```python
from build123d import *

# Parameters (mm, degrees)
SKETCH1_R           = 0.5
BOSS_EXTRUDE1_DEPTH = 3
SKETCH3_R           = 4.5
SKETCH3_R_2         = 2.5
BOSS_EXTRUDE2_DEPTH = 5
SKETCH4_R           = 3
CUT_EXTRUDE1_DEPTH  = 3


with BuildPart() as part:
    # Sketch1 → Boss-Extrude1 (new body)
    with BuildSketch(Plane(origin=(0, 0, 0), x_dir=(1, 0, 0), z_dir=(0, 1, 0))):
        with BuildLine():
            Line((0, 6.5), (29, 4))
            ThreePointArc((29, 4), (33, 0), (29, -4))
            Line((29, -4), (0, -6.5))
            ThreePointArc((0, -6.5), (-6.5, 0), (0, 6.5))
        make_face()
        with Locations(Location((14.5, 0, 0), (0, 0, 270))):
            Circle(SKETCH1_R, mode=Mode.SUBTRACT)
        with Locations(Location((17.5, 0, 0), (0, 0, 270))):
            Circle(SKETCH1_R, mode=Mode.SUBTRACT)
        with Locations(Location((20.5, 0, 0), (0, 0, 270))):
            Circle(SKETCH1_R, mode=Mode.SUBTRACT)
        with Locations(Location((23.5, 0, 0), (0, 0, 270))):
            Circle(SKETCH1_R, mode=Mode.SUBTRACT)
        with Locations(Location((26.5, 0, 0), (0, 0, 270))):
            Circle(SKETCH1_R, mode=Mode.SUBTRACT)
        with Locations(Location((29.5, 0, 0), (0, 0, 270))):
            Circle(SKETCH1_R, mode=Mode.SUBTRACT)
    extrude(amount=BOSS_EXTRUDE1_DEPTH)

    # Sketch3 → Boss-Extrude2 (add)
    with BuildSketch(Plane.XZ):
        with Locations(Location((0, 0, 0), (0, 0, 90))):
            Circle(SKETCH3_R)
        with Locations(Location((0, 0, 0), (0, 0, 270))):
            Circle(SKETCH3_R_2, mode=Mode.SUBTRACT)
    extrude(amount=BOSS_EXTRUDE2_DEPTH)

    # Sketch4 → Cut-Extrude1 (cut)
    with BuildSketch(Plane(origin=(0, 3, 0), x_dir=(1, 0, 0), z_dir=(0, 1, 0))):
        with Locations(Location((0, 0, 0), (0, 0, 270))):
            Circle(SKETCH4_R)
    extrude(amount=-CUT_EXTRUDE1_DEPTH, mode=Mode.SUBTRACT)


solid = part.part
```
Source: CAD feature listing. Evaluate the final solid. Frame: model axes, mm. A direction names the side the tool comes from. Coordinates: 2 decimals unless noted, no trailing zeros. Order: outer loops, then holes, each group sorted by start corner. A loop starts at its lowest first (then second) coordinate and runs counter-clockwise, first axis right, second up. Notation, with made-up numbers: (16.5, 79) - (70.5, 79) arc R18 ccw to (70.5, 97) - close; hole circle Ø3 at (55, 43.5). An arc over 180 degrees is marked (long way). One line per item, written item: value.
1) Contact query for flat-ended pins moving along their axis: pin 1 (2 mm diameter, centred on x = 21, y = 1, fed in from -Z); pin 2 (3 mm diameter, centred on y = -0.5, z = -2.5, fed in from +X); pin 3 (5.5 mm diameter, centred on x = 0, z = 0, fed in from +Y). Output: stop coordinate, or through.
Computed values:
pin 1: stops at z = -4.78
pin 2: stops at x = 32.85
pin 3: stops at y = 0
2) Cut plane B-B on y = 2. Output: boundary loops of the cut face in (x, z), plus the area to 3 significant figures.
Computed values:
outline: (0, -6.5) - (29, -4) arc R4 ccw to (29, 4) - (0, 6.5) arc R6.5 ccw to start; hole circle Ø6 at (0, 0); hole circle Ø1 at (14.5, 0); hole circle Ø1 at (17.5, 0); hole circle Ø1 at (20.5, 0); hole circle Ø1 at (23.5, 0); hole circle Ø1 at (26.5, 0); hole circle Ø1 at (29.5, 0)
area: 363 mm^2
3) Cut plane A-A on x = 14.5. Output: boundary loops of the cut face in (y, z).
Computed values:
outline: (0, -5.25) - (3, -5.25) - (3, -0.5) - (0, -0.5) - close; (0, 0.5) - (3, 0.5) - (3, 5.25) - (0, 5.25) - close
4) Mould query, pull axis X, two halves, no side actions, for faces 1 (the face through (21, 1, 0)), 2 (the face through (-6.5, 1.5, 0.1)), 3 (the face through (13.5, 0, -0.1)). Classes: released by +X, released by -X, zero draft, split by the parting line, or undercut.
Computed values:
face 1: undercut
face 2: released by -X
face 3: zero draft
5) Cut plane C-C on z = 0. State how many separate pieces and enclosed holes the cut face has, plus the area to 4 significant figures.
Computed values:
separate pieces: 8
enclosed holes: 0
area: 102.5 mm^2
6) Reachability of faces 4 (the face through (0.9, 1.52, 2.86)), 5 (the face through (24, 1, 0)), 6 (the face through (-1.352, -2.465, 4.292)) from +Z, -Z, +X, -X, +Y, -Y: full face, straight path, thin tool, end or side. Return the list, or none.
Computed values:
face 4: +Y
face 5: +Y, -Y
face 6: -Y
7) Ray query, line 1 (X direction, y = -0.95, z = 0); line 2 (Y direction, x = 9.5, z = -5); line 3 (X direction, y = -1.5, z = -1.25). Return the intervals inside material, ascending. Write a range as [from, to].
Computed values:
line 1: x = [-4.5, -2.5], [2.5, 4.5]
line 2: y = [0, 3]
line 3: x = [-4.32, -2.17], [2.17, 4.32]
8) Cut plane D-D on x = 26.5. Output: boundary loops of the cut face in (y, z), plus the area to 3 significant figures.
Computed values:
outline: (0, -4.22) - (3, -4.22) - (3, -0.5) - (0, -0.5) - close; (0, 0.5) - (3, 0.5) - (3, 4.22) - (0, 4.22) - close
area: 22.3 mm^2
